Source: CAD feature listing. Evaluate the final solid. Frame: model axes, mm. Coordinates: 2 decimals unless noted, no trailing zeros. Order: outer loops, then holes, each group sorted by start corner. A loop starts at its lowest first (then second) coordinate and runs counter-clockwise, first axis right, second up. Notation, with made-up numbers: (16, 48.25) - (36, 48.25) arc R21 cw to (36, 76.25) - close; hole circle Ø5 at (54.25, 36). An arc over 180 degrees is marked (long way). One line per question, with ' | ' between items. Start each with the question number.
(1) Section B-B (y = -2.2). Return the cut outline in (x, z) (3 decimals), then the cut area to 3 significant figures.
(2) Section C-C (y = 0.35). Return the cut outline in (x, z) (3 decimals).
(3) Line query: line 1 along X through (y, z) = (-1.95, -2); line 2 along X through (y, z) = (1.65, -2.25); line 3 along Z through (x, y) = (-0.75, -1.65) (3 decimals). Output: solid intervals per line, ascending.
(4) Draft query along X for faces 1 (the flat face through (-3.832, 0.035, -2.254)), 2 (the flat face through (0, 0, 4.445)), 3 (the cylindrical face through (-3.05, -0.04, 1.26)). Return one class per face: +X half, -X half, draft (parallel to the pull), parting line (faces both ways), or undercut.
(5) Section A-A (x = 0). Return the cut outline in (y, z) (3 decimals), then the cut area to 3 significant figures.
from build123d import *

# Parameters (mm, degrees)
BOSS_EXTRUDE1_DEPTH = 2.54
HOLE1_D             = 6.604


with BuildPart() as part:
    # Sketch2 → Boss-Extrude1 (new, symmetric)
    with BuildSketch(Plane(origin=(0, 0, 0), x_dir=(1, 0, 0), z_dir=(0, 1, 0))):
        Polygon((5.132643893, 0), (2.566321947, 4.445), (-2.566321947, 4.445), (-5.132643893, 0), (-2.566321947, -4.445), (2.566321947, -4.445), align=None)
    extrude(amount=BOSS_EXTRUDE1_DEPTH, both=True)

    # Sketch3 → Cut-Revolve1 (revolve, cut)
    with BuildSketch(Plane.XY, mode=Mode.PRIVATE) as cut_revolve1_sk:
        Polygon((4.370643893, 2.54), (5.132643893, 2.54), (5.132643893, 1.778), align=None)
    cut_revolve1 = revolve(cut_revolve1_sk.sketch.rotate(Axis((0, 0, 0), (0, 1, 0)), 90), axis=Axis((0, 0, 0), (0, 1, 0)), mode=Mode.SUBTRACT)

    # Hole1 (through all)
    with Locations(Plane(origin=(0, 2.54, 0), x_dir=(1, 0, 0), z_dir=(0, 1, 0))):
        with Locations((0, 0)):
            Hole(HOLE1_D / 2)

    # Mirror1: Cut-Revolve1 across plane
    add(cut_revolve1.mirror(Plane.ZX), mode=Mode.SUBTRACT)


solid = part.part
Response values:
1) outline: (-4.629, -0.872) - (-3.07, -3.573) arc R4.711 ccw to (-1.56, -4.445) - (1.56, -4.445) arc R4.711 ccw to (3.07, -3.573) - (4.629, -0.872) arc R4.711 ccw to (4.629, 0.872) - (3.07, 3.573) arc R4.711 ccw to (1.56, 4.445) - (-1.56, 4.445) arc R4.711 ccw to (-3.07, 3.573) - (-4.629, 0.872) arc R4.711 ccw to start; hole circle Ø6.604 at (0, 0) | area: 32.1 mm²
2) outline: (-5.133, 0) - (-2.566, -4.445) - (2.566, -4.445) - (5.133, 0) - (2.566, 4.445) - (-2.566, 4.445) - close; hole circle Ø6.604 at (0, 0)
3) line 1: x = -3.98 to -2.63, 2.63 to 3.98 | line 2: x = -3.83 to -2.42, 2.42 to 3.83 | line 3: z = -4.445 to -3.216, 3.216 to 4.445
4) face 1: -X half | face 2: draft | face 3: undercut
5) outline: (-2.54, -4.371) - (-2.466, -4.445) - (2.466, -4.445) - (2.54, -4.371) - (2.54, -3.302) - (-2.54, -3.302) - close; (-2.54, 3.302) - (2.54, 3.302) - (2.54, 4.371) - (2.466, 4.445) - (-2.466, 4.445) - (-2.54, 4.371) - close | area: 11.6 mm²
